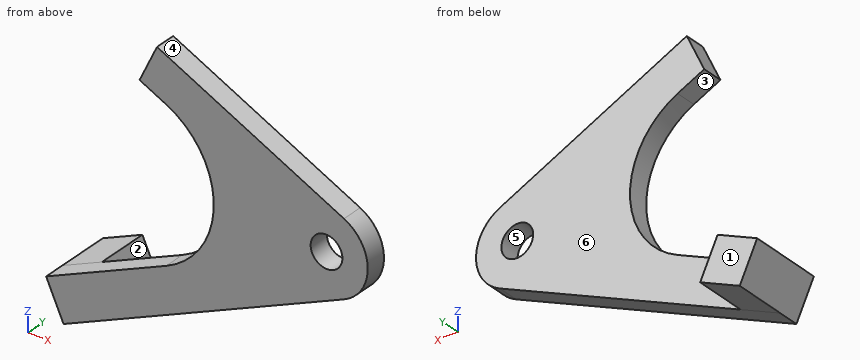
```python
from build123d import *

# Parameters (mm, degrees)
F0_R     = 1.9558
F1_DEPTH = 2.54
F3_DEPTH = 6.35


with BuildPart() as f1:
    # F0 (on Front) → F1 (new body)
    with BuildSketch(Plane.XZ):
        with BuildLine():
            ThreePointArc((2.146901, -4.604044), (5.08, 0), (2.146901, 4.604044))
            Line((2.146901, 4.604044), (-20.873317, 15.338547))
            Line((-20.873317, 15.338547), (-23.020218, 10.734504))
            Line((-23.020218, 10.734504), (-19.746807, 9.208087))
            ThreePointArc((-19.746807, 9.208087), (-13.880608, 0), (-19.746807, -9.208087))
            Line((-19.746807, -9.208087), (-34.530327, -16.101756))
            Line((-34.530327, -16.101756), (-32.383426, -20.705799))
            Line((-32.383426, -20.705799), (2.146901, -4.604044))
        make_face()
        Circle(F0_R, mode=Mode.SUBTRACT)
    extrude(amount=-F1_DEPTH)

    # F2 (on face) → F3 (join)
    with BuildSketch(Plane(origin=(0, 2.54, 0), x_dir=(-1, 0, 0), z_dir=(0, 1, 0))):
        Polygon((32.383426, -20.705799), (34.530327, -16.101756), (29.658666, -13.830063), (27.511766, -18.434107), align=None)
    extrude(amount=F3_DEPTH)


solid = f1.part
```
Geometry check sheet. Reference: the model listing, model coordinates, mm. Face numbers are marked on the shaded views. A direction names the side the tool comes from. Round coordinates to 2 decimals unless told otherwise and drop trailing zeros. Order: outer loops, then holes, each group sorted by start corner. A loop starts at its lowest first (then second) coordinate and runs counter-clockwise, first axis right, second up. Notation, with made-up numbers: (-0.5, 54) - (33.5, 54) arc R33 cw to (33.5, 85) - close; hole circle Ø5 at (66, 31.25). An arc over 180 degrees is marked (long way). Use a Markdown table: item, result. Add a question column.
(1) Sectioned sample at D-D, the plane y = 7. Enter the section's corners in (x, z), and give its area (3 significant figures).
(2) Depth check by flat-ended pin: pin 1 (1 mm diameter, centred on x = -7.5, z = 3, fed in from +Y). Enter the tip coordinate at first touch or a pass-through.
(3) Tool access check on the marked faces 1, 2 and 3. Record the directions out of +Z, -Z, +X, -X, +Y, -Y that give a thin tool (end or side, any length) a straight path to the whole face; none if there is none.
(4) Release check for a two-part mould opening along X. For the marked faces 4, 5 and 6 record: pulls with the +X half, pulls with the -X half, needs draft (parallel to the pull), parting line crosses it, or undercut.
(5) Sectioned sample at A-A, the plane z = 0. Enter the section's corners in (x, y).
(6) Sectioned sample at B-B, the plane x = -18. Enter the section's corners in (y, z).
(7) Material ranges on line 1 along Y through (x, z) = (-17.5, 13.5); line 2 along Z through (x, y) = (0, 0.85); line 3 along Z through (x, y) = (-2, 1), recorded low to high. Write a range as [from, to].
(8) Sectioned sample at C-C, the plane y = 1.5. Enter the section's corners in (x, z), and give its area (3 significant figures).
Answers below:
| question | item | result |
|---|---|---|
| 1 | outline | (-34.53, -16.1) - (-32.38, -20.71) - (-27.51, -18.43) - (-29.66, -13.83) - close |
| 1 | area | 27.3 mm² |
| 2 | pin 1 | y = 2.54 |
| 3 | face 1 | +Z, -Z, +X, -X, +Y |
| 3 | face 2 | +Z, +X, +Y |
| 3 | face 3 | -X, +Y, -Y |
| 4 | face 4 | pulls with the +X half |
| 4 | face 5 | undercut |
| 4 | face 6 | needs draft |
| 5 | outline | (-13.88, 0) - (-1.96, 0) - (-1.96, 2.54) - (-13.88, 2.54) - close; (1.96, 0) - (5.08, 0) - (5.08, 2.54) - (1.96, 2.54) - close |
| 6 | outline | (0, -14) - (2.54, -14) - (2.54, -8.17) - (0, -8.17) - close; (0, 8.17) - (2.54, 8.17) - (2.54, 14) - (0, 14) - close |
| 7 | line 1 | [0, 2.54] |
| 7 | line 2 | [-5.61, -1.96], [1.96, 5.61] |
| 7 | line 3 | [-6.54, 6.54] |
| 8 | outline | (-34.53, -16.1) - (-32.38, -20.71) - (2.15, -4.6) arc R5.08 ccw to (2.15, 4.6) - (-20.87, 15.34) - (-23.02, 10.73) - (-19.75, 9.21) arc R10.16 cw to (-19.75, -9.21) - close; hole circle Ø3.91 at (0, 0) |
| 8 | area | 444 mm² |
